from build123d import *
from OCP.BRepFilletAPI import BRepFilletAPI_MakeChamfer
from build123d.topology import SkipClean

# Parameters (mm, degrees)
SKETCH1_R                      = 158.75
BOSS_EXTRUDE1_DEPTH            = 3.175
BOSS_EXTRUDE2_START            = 26.9875
BOSS_EXTRUDE2_DEPTH            = 26.9875
CHAMFER1_SIZE                  = 26.9875
CHAMFER1_SIZE_2                = 12.7
CBORE_FOR_M3_SHCS1_D           = 3.4
CBORE_FOR_M3_SHCS1_CBORE_D     = 6
CBORE_FOR_M3_SHCS1_CBORE_DEPTH = 3
CIRPATTERN1_COUNT              = 6
CHAMFER1_OF_CIRPATTERN1_SIZE   = 26.9875
CHAMFER1_OF_CIRPATTERN1_SIZE_2 = 12.7
CUT_EXTRUDE1_DEPTH             = 3.175
SKETCH8_W                      = 86
SKETCH8_H                      = 54
CUT_EXTRUDE2_DEPTH             = 1.27
FILLET1_R                      = 2
CUT_EXTRUDE4_DEPTH             = 1.27
CUT_EXTRUDE3_DEPTH             = 26.9875
BOSS_EXTRUDE3_DEPTH            = 3.175
CHAMFER2_SIZE                  = 2


with BuildPart() as part:
    # Sketch1 → Boss-Extrude1 (new body)
    with BuildSketch(Plane.XY):
        Circle(SKETCH1_R)
    extrude(amount=BOSS_EXTRUDE1_DEPTH)

    # Sketch9 → Boss-Extrude2 (add)
    with SkipClean():  # the faces are left unmerged after this step: merging them gives an invalid solid
        with BuildSketch(Plane(origin=(0, 0, 0), x_dir=(-1, 0, 0), z_dir=(0, 0, -1)).offset(BOSS_EXTRUDE2_START)):
            with BuildLine():
                Line((-27.566648205, 156.338230791), (-26.463982276, 150.084701559))
                ThreePointArc((-26.463982276, 150.084701559), (0, 152.4), (26.463982276, 150.084701559))
                Line((26.463982276, 150.084701559), (27.566648205, 156.338230791))
                ThreePointArc((27.566648205, 156.338230791), (0, 158.75), (-27.566648205, 156.338230791))
            make_face()
        boss_extrude2 = extrude(amount=-BOSS_EXTRUDE2_DEPTH)

    # Chamfer1
    chamfer1_edges_1 = [part.edges().sort_by_distance(p)[0] for p in [
        (27.015315241, 153.211466175, -26.9875),
    ]]
    chamfer1_side_1 = [part.faces().sort_by_distance(p)[0] for p in [
        (27.015315241, 153.211466175, -26.7335),
    ]]
    chamfer1_edges_2 = [part.edges().sort_by_distance(p)[0] for p in [
        (-27.015315241, 153.211466175, -26.9875),
    ]]
    chamfer1_side_2 = [part.faces().sort_by_distance(p)[0] for p in [
        (-27.015315241, 153.211466175, -26.7335),
    ]]
    chamfer1 = BRepFilletAPI_MakeChamfer(part.part.solid().wrapped)
    for e in chamfer1_edges_1:
        chamfer1.Add(CHAMFER1_SIZE - 0.0001, CHAMFER1_SIZE_2 - 0.0001, e.wrapped, chamfer1_side_1[0].wrapped)
    for e in chamfer1_edges_2:
        chamfer1.Add(CHAMFER1_SIZE - 0.0001, CHAMFER1_SIZE_2 - 0.0001, e.wrapped, chamfer1_side_2[0].wrapped)
    add(Compound.cast(chamfer1.Shape()), mode=Mode.REPLACE)  # a hair under: the kernel refuses the full size

    # CBORE for M3 SHCS1 (through all)
    with Locations(Plane.XY.offset(3.175)):
        with Locations((0, 155.575)):
            cbore_for_m3_shcs1 = CounterBoreHole(CBORE_FOR_M3_SHCS1_D / 2, CBORE_FOR_M3_SHCS1_CBORE_D / 2, CBORE_FOR_M3_SHCS1_CBORE_DEPTH)

    # CirPattern1: Boss-Extrude2, CBORE for M3 SHCS1 ×6 about axis
    cirpattern1_axis = Axis((0, 0, 0), (0, 0, 1))
    add([boss_extrude2.rotate(cirpattern1_axis, i * 360 / CIRPATTERN1_COUNT) for i in range(1, CIRPATTERN1_COUNT)])
    add([cbore_for_m3_shcs1.rotate(cirpattern1_axis, i * 360 / CIRPATTERN1_COUNT) for i in range(1, CIRPATTERN1_COUNT)], mode=Mode.SUBTRACT)

    # Chamfer1 of CirPattern1
    chamfer1_of_cirpattern1_edges_1 = [part.edges().sort_by_distance(p)[0] for p in [
        (-119.177364238, 100.001682377, -26.9875),
    ]]
    chamfer1_of_cirpattern1_side_1 = [part.faces().sort_by_distance(p)[0] for p in [
        (-119.177364238, 100.001682377, -26.7335),
    ]]
    chamfer1_of_cirpattern1_edges_2 = [part.edges().sort_by_distance(p)[0] for p in [
        (-146.192679479, 53.209783798, -26.9875),
    ]]
    chamfer1_of_cirpattern1_side_2 = [part.faces().sort_by_distance(p)[0] for p in [
        (-146.192679479, 53.209783798, -26.7335),
    ]]
    chamfer1_of_cirpattern1_edges_3 = [part.edges().sort_by_distance(p)[0] for p in [
        (-146.192679479, -53.209783798, -26.9875),
    ]]
    chamfer1_of_cirpattern1_side_3 = [part.faces().sort_by_distance(p)[0] for p in [
        (-146.192679479, -53.209783798, -26.7335),
    ]]
    chamfer1_of_cirpattern1_edges_4 = [part.edges().sort_by_distance(p)[0] for p in [
        (-119.177364238, -100.001682377, -26.9875),
    ]]
    chamfer1_of_cirpattern1_side_4 = [part.faces().sort_by_distance(p)[0] for p in [
        (-119.177364238, -100.001682377, -26.7335),
    ]]
    chamfer1_of_cirpattern1_edges_5 = [part.edges().sort_by_distance(p)[0] for p in [
        (-27.015315241, -153.211466175, -26.9875),
    ]]
    chamfer1_of_cirpattern1_side_5 = [part.faces().sort_by_distance(p)[0] for p in [
        (-27.015315241, -153.211466175, -26.7335),
    ]]
    chamfer1_of_cirpattern1_edges_6 = [part.edges().sort_by_distance(p)[0] for p in [
        (27.015315241, -153.211466175, -26.9875),
    ]]
    chamfer1_of_cirpattern1_side_6 = [part.faces().sort_by_distance(p)[0] for p in [
        (27.015315241, -153.211466175, -26.7335),
    ]]
    chamfer1_of_cirpattern1_edges_7 = [part.edges().sort_by_distance(p)[0] for p in [
        (119.177364238, -100.001682377, -26.9875),
    ]]
    chamfer1_of_cirpattern1_side_7 = [part.faces().sort_by_distance(p)[0] for p in [
        (119.177364238, -100.001682377, -26.7335),
    ]]
    chamfer1_of_cirpattern1_edges_8 = [part.edges().sort_by_distance(p)[0] for p in [
        (146.192679479, -53.209783798, -26.9875),
    ]]
    chamfer1_of_cirpattern1_side_8 = [part.faces().sort_by_distance(p)[0] for p in [
        (146.105806362, -53.448465724, -26.9875),
    ]]
    chamfer1_of_cirpattern1_edges_9 = [part.edges().sort_by_distance(p)[0] for p in [
        (146.192679479, 53.209783798, -26.9875),
    ]]
    chamfer1_of_cirpattern1_side_9 = [part.faces().sort_by_distance(p)[0] for p in [
        (146.192679479, 53.209783798, -26.7335),
    ]]
    chamfer1_of_cirpattern1_edges_10 = [part.edges().sort_by_distance(p)[0] for p in [
        (119.177364238, 100.001682377, -26.9875),
    ]]
    chamfer1_of_cirpattern1_side_10 = [part.faces().sort_by_distance(p)[0] for p in [
        (119.177364238, 100.001682377, -26.7335),
    ]]
    chamfer1_of_cirpattern1 = BRepFilletAPI_MakeChamfer(part.part.solid().wrapped)
    for e in chamfer1_of_cirpattern1_edges_1:
        chamfer1_of_cirpattern1.Add(CHAMFER1_OF_CIRPATTERN1_SIZE - 0.0001, CHAMFER1_OF_CIRPATTERN1_SIZE_2 - 0.0001, e.wrapped, chamfer1_of_cirpattern1_side_1[0].wrapped)
    for e in chamfer1_of_cirpattern1_edges_2:
        chamfer1_of_cirpattern1.Add(CHAMFER1_OF_CIRPATTERN1_SIZE - 0.0001, CHAMFER1_OF_CIRPATTERN1_SIZE_2 - 0.0001, e.wrapped, chamfer1_of_cirpattern1_side_2[0].wrapped)
    for e in chamfer1_of_cirpattern1_edges_3:
        chamfer1_of_cirpattern1.Add(CHAMFER1_OF_CIRPATTERN1_SIZE - 0.0001, CHAMFER1_OF_CIRPATTERN1_SIZE_2 - 0.0001, e.wrapped, chamfer1_of_cirpattern1_side_3[0].wrapped)
    for e in chamfer1_of_cirpattern1_edges_4:
        chamfer1_of_cirpattern1.Add(CHAMFER1_OF_CIRPATTERN1_SIZE - 0.0001, CHAMFER1_OF_CIRPATTERN1_SIZE_2 - 0.0001, e.wrapped, chamfer1_of_cirpattern1_side_4[0].wrapped)
    for e in chamfer1_of_cirpattern1_edges_5:
        chamfer1_of_cirpattern1.Add(CHAMFER1_OF_CIRPATTERN1_SIZE - 0.0001, CHAMFER1_OF_CIRPATTERN1_SIZE_2 - 0.0001, e.wrapped, chamfer1_of_cirpattern1_side_5[0].wrapped)
    for e in chamfer1_of_cirpattern1_edges_6:
        chamfer1_of_cirpattern1.Add(CHAMFER1_OF_CIRPATTERN1_SIZE - 0.0001, CHAMFER1_OF_CIRPATTERN1_SIZE_2 - 0.0001, e.wrapped, chamfer1_of_cirpattern1_side_6[0].wrapped)
    for e in chamfer1_of_cirpattern1_edges_7:
        chamfer1_of_cirpattern1.Add(CHAMFER1_OF_CIRPATTERN1_SIZE - 0.0001, CHAMFER1_OF_CIRPATTERN1_SIZE_2 - 0.0001, e.wrapped, chamfer1_of_cirpattern1_side_7[0].wrapped)
    for e in chamfer1_of_cirpattern1_edges_8:
        chamfer1_of_cirpattern1.Add(CHAMFER1_OF_CIRPATTERN1_SIZE_2 - 0.0001, CHAMFER1_OF_CIRPATTERN1_SIZE - 0.0001, e.wrapped, chamfer1_of_cirpattern1_side_8[0].wrapped)
    for e in chamfer1_of_cirpattern1_edges_9:
        chamfer1_of_cirpattern1.Add(CHAMFER1_OF_CIRPATTERN1_SIZE - 0.0001, CHAMFER1_OF_CIRPATTERN1_SIZE_2 - 0.0001, e.wrapped, chamfer1_of_cirpattern1_side_9[0].wrapped)
    for e in chamfer1_of_cirpattern1_edges_10:
        chamfer1_of_cirpattern1.Add(CHAMFER1_OF_CIRPATTERN1_SIZE - 0.0001, CHAMFER1_OF_CIRPATTERN1_SIZE_2 - 0.0001, e.wrapped, chamfer1_of_cirpattern1_side_10[0].wrapped)
    add(Compound.cast(chamfer1_of_cirpattern1.Shape()), mode=Mode.REPLACE)  # a hair under: the kernel refuses the full size

    # Sketch7 → Cut-Extrude1 (cut)
    with BuildSketch(Plane.XY.offset(3.175)):
        with BuildLine():
            Line((-1.5875, 132.368516096), (-1.5875, 135.255))
            ThreePointArc((-1.5875, 135.255), (0, 136.8425), (1.5875, 135.255))
            Line((1.5875, 135.255), (1.5875, 132.368516096))
            ThreePointArc((1.5875, 132.368516096), (0, 125.095), (-1.5875, 132.368516096))
        make_face()
    extrude(amount=-CUT_EXTRUDE1_DEPTH, mode=Mode.SUBTRACT)

    # Sketch8 → Cut-Extrude2 (cut)
    with BuildSketch(Plane.XY.offset(3.175)):
        with Locations((0, -77.775)):
            Rectangle(SKETCH8_W, SKETCH8_H)
    extrude(amount=-CUT_EXTRUDE2_DEPTH, mode=Mode.SUBTRACT)

    # Fillet1
    fillet1_edges = [part.edges().sort_by_distance(p)[0] for p in [
        (-43, -104.775, 2.54),
        (-43, -50.775, 2.54),
        (43, -50.775, 2.54),
        (43, -104.775, 2.54),
    ]]
    fillet(fillet1_edges, radius=FILLET1_R)

    # Sketch13 → Cut-Extrude4 (cut)
    with BuildSketch(Plane.XY.offset(3.175)):
        with BuildLine():
            Line((-43.5, -52.775), (-43.5, -102.775))
            ThreePointArc((-43.5, -102.775), (-42.767766953, -104.542766953), (-41, -105.275))
            Line((-41, -105.275), (41, -105.275))
            ThreePointArc((41, -105.275), (42.767766953, -104.542766953), (43.5, -102.775))
            Line((43.5, -102.775), (43.5, -52.775))
            ThreePointArc((43.5, -52.775), (42.767766953, -51.007233047), (41, -50.275))
            Line((41, -50.275), (-41, -50.275))
            ThreePointArc((-41, -50.275), (-42.767766953, -51.007233047), (-43.5, -52.775))
        make_face()
    extrude(amount=-CUT_EXTRUDE4_DEPTH, mode=Mode.SUBTRACT)

    # Sketch10 → Cut-Extrude3 (cut)
    with BuildSketch(Plane(origin=(0, 0, -26.9875), x_dir=(-1, 0, 0), z_dir=(0, 0, -1))):
        with BuildLine():
            ThreePointArc((-144.354417642, -66.055768917), (-142.016041239, -70.943685629), (-139.512216635, -75.748953191))
            Line((-139.512216635, -75.748953191), (-133.93172797, -72.718995064))
            ThreePointArc((-133.93172797, -72.718995064), (-136.221318638, -68.333830192), (-138.367379277, -63.876665161))
            Line((-138.367379277, -63.876665161), (-144.354417642, -66.055768917))
        make_face()
        with BuildLine():
            Line((-129.942361048, -79.628781263), (-135.356626091, -82.946647149))
            ThreePointArc((-135.356626091, -82.946647149), (-132.447054613, -87.517656643), (-129.38318277, -91.986708368))
            Line((-129.38318277, -91.986708368), (-124.502504377, -87.891332929))
            ThreePointArc((-124.502504377, -87.891332929), (-127.289492203, -83.804207381), (-129.942361048, -79.628781263))
        make_face()
        with BuildLine():
            ThreePointArc((-149.17620355, -54.295697753), (-146.883052844, -60.224009226), (-144.354417642, -66.055768917))
            Line((-144.354417642, -66.055768917), (-138.367379277, -63.876665161))
            ThreePointArc((-138.367379277, -63.876665161), (-140.910852211, -58.05076855), (-143.209155408, -52.123869843))
            Line((-143.209155408, -52.123869843), (-149.17620355, -54.295697753))
        make_face()
        with BuildLine():
            Line((-124.502504377, -87.891332929), (-129.38318277, -91.986708368))
            ThreePointArc((-129.38318277, -91.986708368), (-125.597048329, -97.092450535), (-121.609555345, -102.042533038))
            Line((-121.609555345, -102.042533038), (-116.745173131, -97.960831716))
            ThreePointArc((-116.745173131, -97.960831716), (-120.728866379, -93.006993408), (-124.502504377, -87.891332929))
        make_face()
    extrude(amount=-CUT_EXTRUDE3_DEPTH, mode=Mode.SUBTRACT)

    # Sketch11 → Boss-Extrude3 (add, symmetric)
    with BuildSketch(Plane(origin=(0, 0, 0), x_dir=(0, 0, -1), z_dir=(1, 0, 0))):
        Polygon((26.9875, 152.4), (0, 152.4), (0, 139.7), align=None)
    extrude(amount=BOSS_EXTRUDE3_DEPTH, both=True)

    # Chamfer2
    chamfer2_edges = [part.edges().sort_by_distance(p)[0] for p in [
        (131.982271537, -76.2, 0),
        (0, -152.4, 0),
        (-131.982271537, -76.2, 0),
        (-131.982271537, 76.2, 0),
        (-14.863359372, 151.673466856, 0),
        (14.863359372, 151.673466856, 0),
        (131.982271537, 76.2, 0),
    ]]
    chamfer(chamfer2_edges, length=CHAMFER2_SIZE)


solid = part.part
For this review, take the finished solid that the model builds, in its own axes (mm). A direction names the side the tool comes from. Give positions to 0.01 mm unless a question says otherwise; leave off trailing zeros. Loops run counter-clockwise (first coordinate to the right, second up) from the corner with the lowest first, then second, coordinate; pieces in that order, holes last. Notation, with made-up numbers: M 51,58.5 L 59,58.5 A31 cw 59,96.5 Z; hole C 28,-15 d10. An arc over 180 degrees is marked long. Put each result on its own line as item: value. Start each with the question number.
(1) Add section B-B, the plane y = 0. Write out the cut boundary in (x, z) (3 decimals), then the cut area to 3 significant figures.
(2) Add section A-A, the plane z = -13. Give the number of separate pieces and of enclosed holes in the cut face, then the cut area to 3 significant figures.
(3) For pin 1 (2.5 mm diameter, centred on x = -134.73, y = -77.79, fed in from +Z); pin 2 (5.5 mm diameter, centred on x = 0, y = -155.575, fed in from +Z) (3 decimals); pin 3 (5 mm diameter, centred on x = 0.5, y = -156.5, fed in from +Z) (3 decimals); pin 4 (10 mm diameter, centred on x = 94.5, y = -39.5, fed in from -Z), all flat-tipped, find the tip position at first contact; note any pin that passes through.
(4) Add section C-C, the plane x = 82. Write out the cut boundary in (y, z) (3 decimals), then the cut area to 3 significant figures.
(5) Machinability: for faces 1 (the flat face through (20.652, -154.201, -13.683)), 2 (the flat face through (3.175, 148, -10)), 3 (the flat face through (-123.306, 95.06, -13.683)), 4 (the flat face through (-1, -77, 1.905)), which of the approach directions +Z, -Z, +X, -X, +Y, -Y give a long, thin tool a straight path to every point of the face, cutting with its end or side? Answer none if there is none.
(6) Wall thickness on L1, parallel to Y at x = 0, z = -16 (3 decimals); L2, parallel to Z at x = 43.5, y = -16 (3 decimals); L3, parallel to Z at x = 25, y = -85 (3 decimals): over which ranges is each line inside the solid? List them lowest first.
(7) The part is to be moulded in two halves that separate along X. For faces 5 (the flat face through (20.672, 154.316, -13.683)), 6 (the flat face through (-2, 2, 3.175)), 7 (the cylindrical face through (-132.16, -75.89, -14.67)), say which applies: +X half, -X half, draft (parallel to the pull), parting line (faces both ways), or undercut.
Result:
1. outline: M -158.75,0 L 158.75,0 L 158.75,3.175 L -158.75,3.175 Z
1. area: 1,010 mm^2
2. separate pieces: 6
2. enclosed holes: 6
2. area: 1,370 mm^2
3. pin 1: passes through
3. pin 2: stops at z = 0.175
3. pin 3: stops at z = 3.175
3. pin 4: stops at z = 0
4. outline: M -135.932,0 L 135.932,0 L 135.932,3.175 L -135.932,3.175 Z
4. area: 863 mm^2
5. face 1: -Z, +X
5. face 2: -Z
5. face 3: -Z, +Y
5. face 4: +Z
6. L1: y = -158.75 to -157.275, -153.875 to -152.4, 147.229 to 153.875, 157.275 to 158.75
6. L2: z = 0 to 3.175
6. L3: z = 0 to 1.905
7. face 5: +X half
7. face 6: draft
7. face 7: undercut
